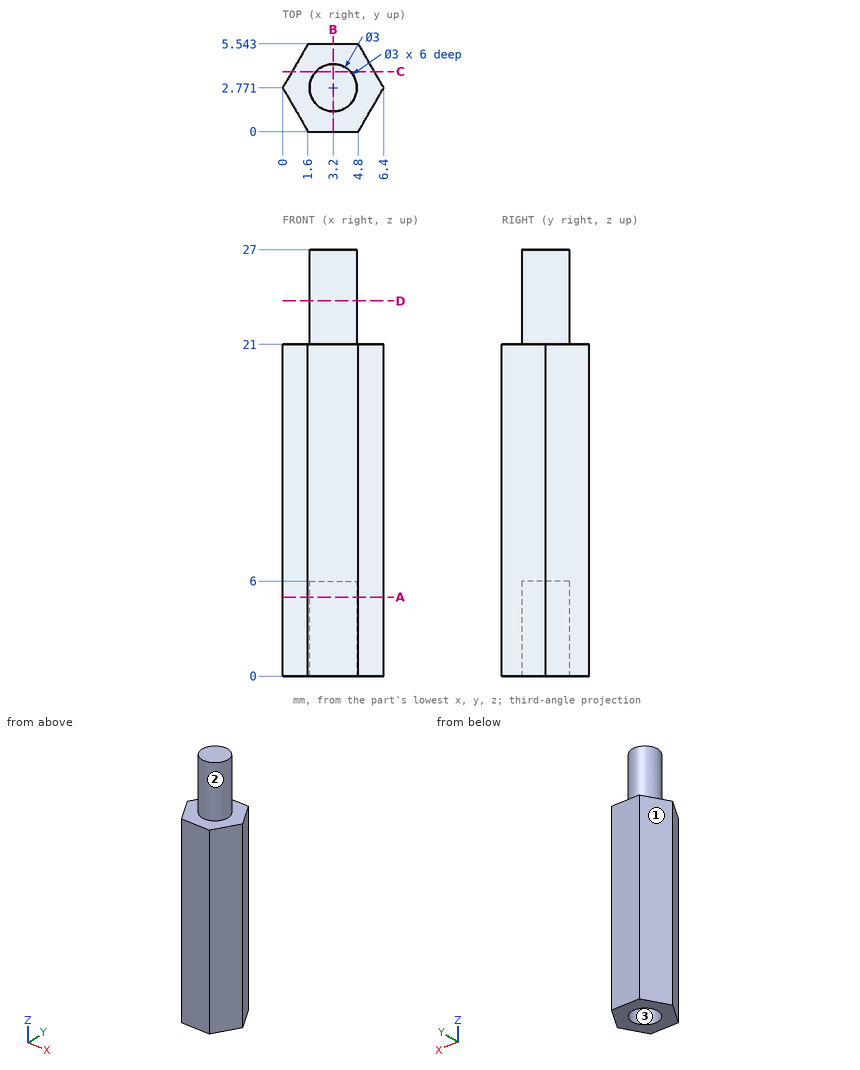
Input: dimensioned drawing with shaded views. Units: mm. Origin: part minimum x, y, z. Coordinates: 2 decimals unless noted, no trailing zeros. Write each loop counter-clockwise with the first axis right and the second up, starting at its lowest first coordinate (ties: lowest second). Pieces come first, ordered by that corner, then holes. Notation, with made-up numbers: (11, 34.25) -> (63, 34.25) arc R23 ccw to (63, 47.25) -> close; hole circle Ø10 at (-6, 78). An arc over 180 degrees is marked (long way). Return JSON: item names as keys, results as strings. Group by question number.
1) Section query C-C, the plane y = 3.8. Return loops of the section in (x, z).
2) Section query B-B, the plane x = 3.2. Return loops of the section in (y, z), plus the area to 3 significant figures.
3) Contact query for flat-ended pins moving along their axis: P1, Ø1, axis at x = 5, z = 18.5, coming from the +Y side; P2, Ø1, axis at x = 2, z = 22.5, coming from the +Y side. Output: stop coordinate, or through.
4) Mould query, pull axis Y, two halves, no side actions, for the marked faces 1, 2 and 3. Classes: +Y half, -Y half, draft (parallel to the pull), parting line (faces both ways), or undercut.
5) Section query A-A, the plane z = 5. Return loops of the section in (x, y).
6) Ray query, line 1 along Y through (x, z) = (3.2, 3.8); line 2 along Z through (x, y) = (2, 1.75); line 3 along Z through (x, y) = (3.25, 1.5). Return the intervals inside material, ascending.
7) Section query D-D, the plane z = 23.75. Return loops of the section in (x, y).
From the geometry:
{
 "1": {"outline": "(0.59, 0) -> (2.11, 0) -> (2.11, 6) -> (4.29, 6) -> (4.29, 0) -> (5.81, 0) -> (5.81, 21) -> (4.29, 21) -> (4.29, 27) -> (2.11, 27) -> (2.11, 21) -> (0.59, 21) -> close"},
 "2": {"outline": "(0, 0) -> (1.27, 0) -> (1.27, 6) -> (4.27, 6) -> (4.27, 0) -> (5.54, 0) -> (5.54, 21) -> (4.27, 21) -> (4.27, 27) -> (1.27, 27) -> (1.27, 21) -> (0, 21) -> close", "area": "116 mm²"},
 "3": {"P1": "y = 5.54", "P2": "y = 4.1"},
 "4": {"face 1": "+Y half", "face 2": "parting line", "face 3": "undercut"},
 "5": {"outline": "(0, 2.77) -> (1.6, 0) -> (4.8, 0) -> (6.4, 2.77) -> (4.8, 5.54) -> (1.6, 5.54) -> close; hole circle Ø3 at (3.2, 2.77)"},
 "6": {"line 1": "0 to 1.27, 4.27 to 5.54", "line 2": "0 to 21", "line 3": "6 to 27"},
 "7": {"outline": "circle Ø3 at (3.2, 2.77)"}
}
